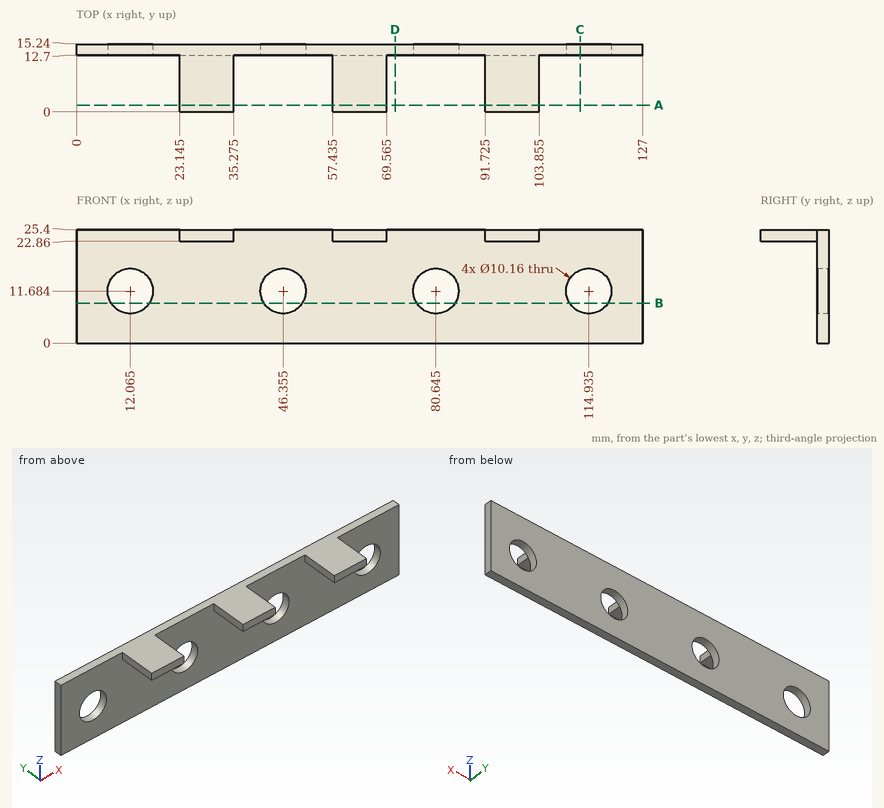
Answer from the drawing. Dimensions are ordinates in mm from the lowest x, y and z of the part. Round coordinates to 2 decimals unless told otherwise and drop trailing zeros. Order: outer loops, then holes, each group sorted by start corner. A loop starts at its lowest first (then second) coordinate and runs counter-clockwise, first axis right, second up. Notation, with made-up numbers: (-15, -7.5) -> (6, -7.5) arc R6 cw to (6, 3.5) -> close; hole circle Ø6 at (-33, 51.5). An arc over 180 degrees is marked (long way). Answer as CSV lines item,"result".
Q1. A cutting plane is placed at C-C on x = 113. Determine the outline of the cut face in (y, z).
Computed values:
outline,"(12.7, 0) -> (15.24, 0) -> (15.24, 6.99) -> (12.7, 6.99) -> close; (12.7, 16.38) -> (15.24, 16.38) -> (15.24, 25.4) -> (12.7, 25.4) -> close"
Q2. A cutting plane is placed at B-B on z = 9. Determine the outline of the cut face in (x, y).
Computed values:
outline,"(0, 12.7) -> (7.75, 12.7) -> (7.75, 15.24) -> (0, 15.24) -> close; (16.38, 12.7) -> (42.04, 12.7) -> (42.04, 15.24) -> (16.38, 15.24) -> close; (50.67, 12.7) -> (76.33, 12.7) -> (76.33, 15.24) -> (50.67, 15.24) -> close; (84.96, 12.7) -> (110.62, 12.7) -> (110.62, 15.24) -> (84.96, 15.24) -> close; (119.25, 12.7) -> (127, 12.7) -> (127, 15.24) -> (119.25, 15.24) -> close"
Q3. Given pin 1 (1.3 mm diameter, centred on y = 7.5, z = 23.5, fed in from +X) (3 decimals); pin 2 (3.5 mm diameter, centred on x = 95, y = 5.5, fed in from -Z); pin 3 (2 mm diameter, centred on y = 6.5, z = 24, fed in from -X) (3 decimals), each flat-ended and moving along its own axis, determine where each tip first touches the part or whether it passes through.
Computed values:
pin 1,"stops at x = 103.855"
pin 2,"stops at z = 22.86"
pin 3,"stops at x = 23.145"
Q4. Consider line 1 (Z direction, x = 33.5, y = 6); line 2 (Y direction, x = 92, z = 6.75). Determine where each line is inside the solid, lowest interval first. Write a range as from..to.
Computed values:
line 1,"z = 22.86..25.4"
line 2,"y = 12.7..15.24"
Q5. A cutting plane is placed at A-A on y = 1.5. Determine the outline of the cut face in (x, z) (3 decimals), plus the area to 3 significant figures.
Computed values:
outline,"(23.145, 22.86) -> (35.275, 22.86) -> (35.275, 25.4) -> (23.145, 25.4) -> close; (57.435, 22.86) -> (69.565, 22.86) -> (69.565, 25.4) -> (57.435, 25.4) -> close; (91.725, 22.86) -> (103.855, 22.86) -> (103.855, 25.4) -> (91.725, 25.4) -> close"
area,"92.4 mm^2"
Q6. A cutting plane is placed at D-D on x = 71.5. Determine the outline of the cut face in (y, z), plus the area to 3 significant figures.
Computed values:
outline,"(12.7, 0) -> (15.24, 0) -> (15.24, 25.4) -> (12.7, 25.4) -> close"
area,"64.5 mm^2"
